Job drawing, mm, ordinate dimensions from the low corner. One solid piece. A direction names the side the tool comes from. Round coordinates to 2 decimals unless told otherwise and drop trailing zeros. Loops run counter-clockwise (first coordinate to the right, second up) from the corner with the lowest first, then second, coordinate; pieces in that order, holes last. Notation, with made-up numbers: M -38.5,-38 L -5.5,-38 A23 cw -5.5,1 Z; hole C -26.75,32.5 d2. An arc over 180 degrees is marked long. Use one line per item in the form item = value.
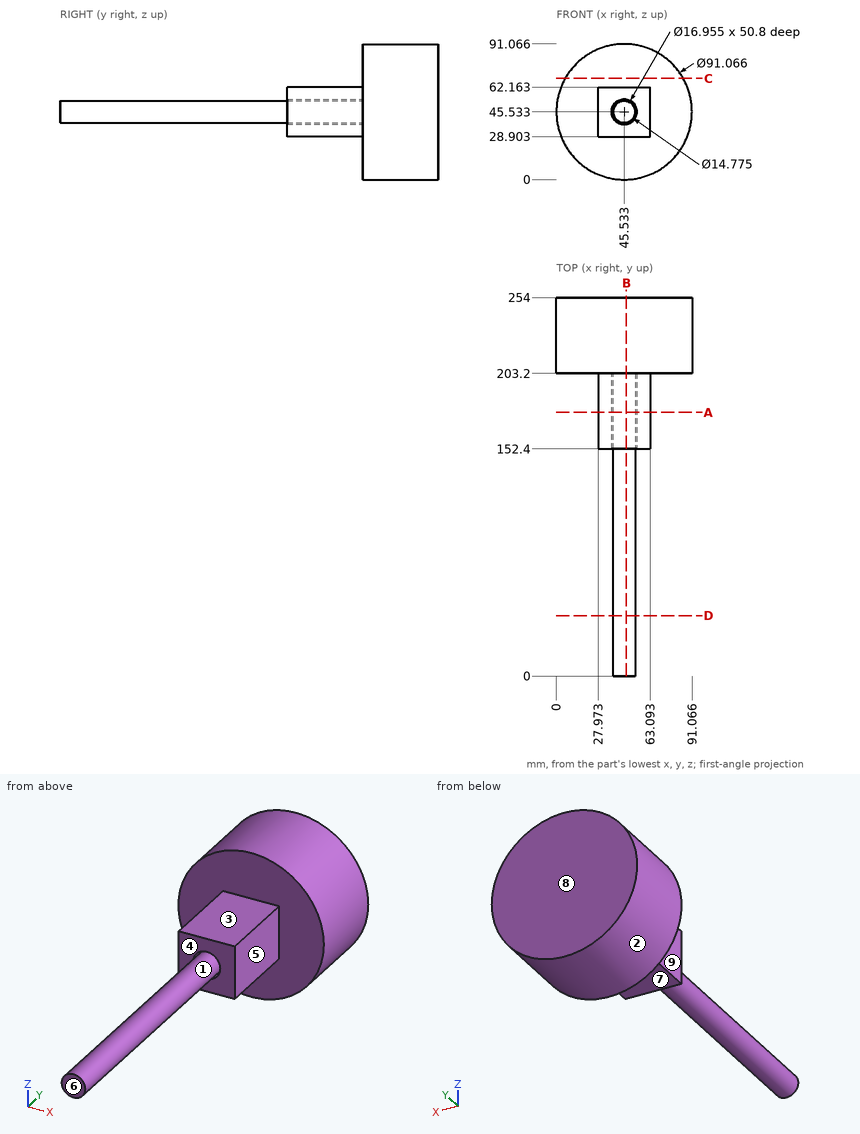
1. Drop flat-ended pins along their axis: P1, Ø10.5, axis at x = 45.5, y = 176, coming from the +Z side; P2, Ø6, axis at y = 173, z = 45, coming from the -X side; P3, Ø4, axis at x = 23, z = 59.5, coming from the -Y side. Give the stop position or say it passes through.
Completed:
P1 = 62.16
P2 = 27.97
P3 = 203.2
2. Cut at C-C on z = 68. Write the cut outline in (x, y).
Completed:
outline = M 5.93,203.2 L 85.14,203.2 L 85.14,254 L 5.93,254 Z
3. Cut at D-D on y = 40.5. Write the cut outline in (x, z) (1 decimal).
Completed:
outline = C 45.5,45.5 d14.8
4. Tool access for the marked faces 5, 6, 7, 8 and 9: list every direction of +Z, -Z, +X, -X, +Y, -Y with a clear straight run to the whole face (end or side of a thin tool).
Completed:
face_5 = +Z, -Z, +X, -Y
face_6 = +Z, -Z, +X, -X, -Y
face_7 = -Z, +X, -X, -Y
face_8 = +Z, -Z, +X, -X, +Y
face_9 = +Z, -Z, -X, -Y
5. Cut at B-B on x = 47. Write the cut outline in (y, z), and give its area (3 significant figures).
Completed:
outline = M 0,38.29 L 203.2,38.29 L 203.2,37.18 L 152.4,37.18 L 152.4,28.9 L 203.2,28.9 L 203.2,0.02 L 254,0.02 L 254,91.04 L 203.2,91.04 L 203.2,62.16 L 152.4,62.16 L 152.4,53.88 L 203.2,53.88 L 203.2,52.77 L 0,52.77 Z
area = 8,410 mm2
6. Probe line 1 along Y through (x, z) = (61, 82); line 2 along X through (y, z) = (177, 36); line 3 along Z through (x, y) = (62, 155.5). List the from-to ranges inside material, lowest first. Write a range as from..to.
Completed:
line_1 = 203.2..254
line_2 = 27.97..63.09
line_3 = 28.9..62.16
7. Cut at A-A on y = 177. Write the cut outline in (x, z) (1 decimal).
Completed:
outline = M 28,28.9 L 63.1,28.9 L 63.1,62.2 L 28,62.2 Z; C 45.5,45.5 d14.8; hole C 45.5,45.5 d17
8. Pull direction Z, two halves, no side cores. Call the marked faces 1, 2, 3 and 4: +Z half, -Z half, draft (parallel to the pull), parting line (faces both ways), or undercut.
Completed:
face_1 = undercut
face_2 = parting line
face_3 = +Z half
face_4 = draft
